Design review of the part shown in the three views and the two pictorial views. Dimensions are in mm from the part's minimum x, y and z. A direction names the side the tool comes from. Round coordinates to 2 decimals unless told otherwise and drop trailing zeros. Loops run counter-clockwise (first coordinate to the right, second up) from the corner with the lowest first, then second, coordinate; pieces in that order, holes last. Notation, with made-up numbers: (38, 57.5) -> (52, 57.5) arc R5 cw to (52, 62.5) -> close; hole circle Ø2 at (65, -39.5). An arc over 180 degrees is marked (long way). One line per question, with ' | ' between items. Start each with the question number.
1. Consider section C-C (z = 396.5). Write out the cut boundary in (x, y), and give its area (3 significant figures).
2. Consider section A-A (y = 626). Write out the cut boundary in (x, z), and give its area (3 significant figures).
3. For pin 1 Ø5 at (x, y) = (315.5, 87) entering from -Z; pin 2 Ø12 at (x, z) = (1541.5, 287.5) entering from -Y; pin 3 Ø10 at (x, y) = (1205, 342.5) entering from +Z; pin 4 Ø23 at (x, z) = (1165.5, 943.5) entering from -Y, all flat-tipped, find the tip position at first contact; note any pin that passes through.
4. For the marked faces 1, 2 and 3, list the 3-axis set-ups (+Z, -Z, +X, -X, +Y, -Y) from which the entire face can be reached by the end or side of a thin tool; tool diameter is ignored.
5. Draft analysis for pull direction Y (two halves, no side actions). For the marked faces 4, 5 and 6, state which applies: pulls with the +Y half, pulls with the -Y half, needs draft (parallel to the pull), parting line crosses it, or undercut.
6. Consider section B-B (x = 1201). Write out the cut boundary in (y, z), and give its area (3 significant figures).
7. Wall thickness on line 1 along Z through (x, y) = (1301, 668.5); line 2 along Z through (x, y) = (906, 74); line 3 along X through (y, z) = (648, 667.5): over which ranges is each line inside the solid? List them lowest first.
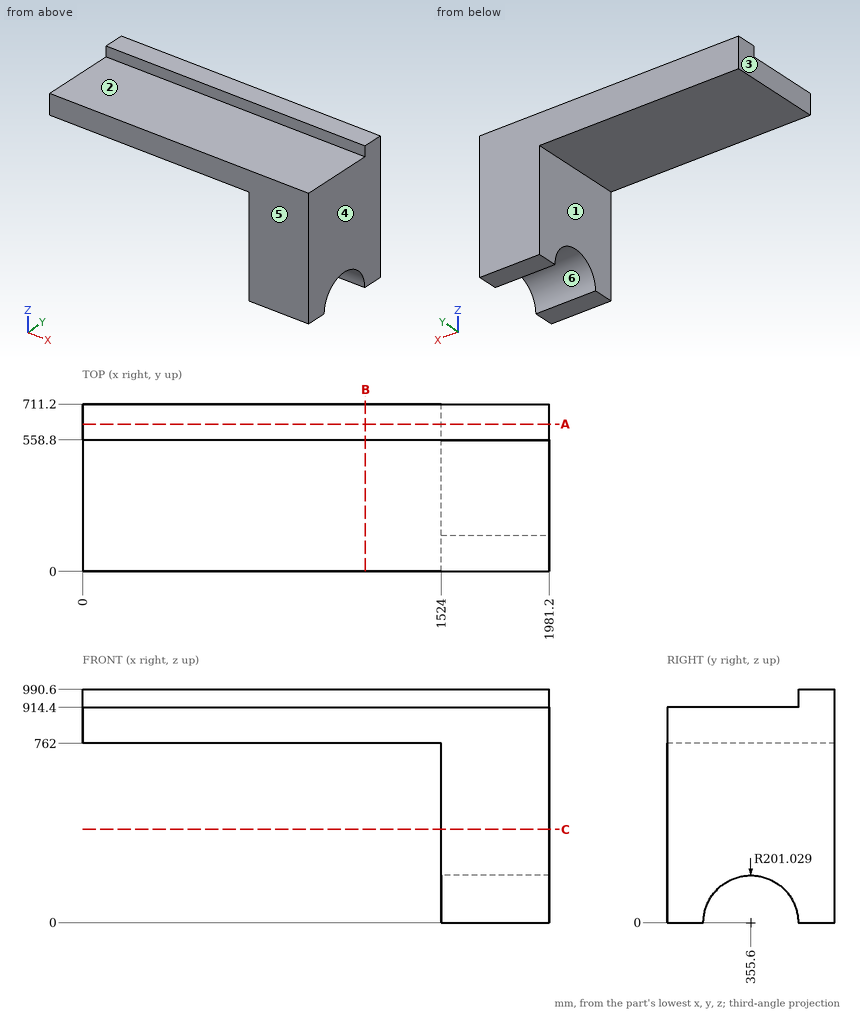
Answer block:
1) outline: (1524, 0) -> (1981.2, 0) -> (1981.2, 711.2) -> (1524, 711.2) -> close | area: 325,000 mm2
2) outline: (0, 762) -> (1524, 762) -> (1524, 0) -> (1981.2, 0) -> (1981.2, 990.6) -> (0, 990.6) -> close | area: 801,000 mm2
3) pin 1: stops at z = 762 | pin 2: stops at y = 0 | pin 3: stops at z = 914.4 | pin 4: stops at y = 558.8
4) face 1: -Z, -X, +Y, -Y | face 2: +Z, +X, -X, -Y | face 3: +Z, -Z, -X, +Y, -Y
5) face 4: needs draft | face 5: pulls with the -Y half | face 6: undercut
6) outline: (0, 762) -> (711.2, 762) -> (711.2, 990.6) -> (558.8, 990.6) -> (558.8, 914.4) -> (0, 914.4) -> close | area: 120,000 mm2
7) line 1: z = 762 to 990.6 | line 2: z = 762 to 914.4 | line 3: x = 1524 to 1981.2
